Input: part model. Units: mm. Frame: model coordinates. Face numbers are marked on the shaded views. Coordinates: 2 decimals unless noted, no trailing zeros. Use a Markdown table: item, result. Add a question column.
1. Line query: L1, parallel to Y at x = 109.5, z = 121.5; L2, parallel to Z at x = 321.5, y = 302; L3, parallel to X at y = 96.5, z = 97.5. Output: solid intervals per line, ascending. Write a range as [from, to].
2. Draft query along Y for the marked faces 1, 2 and 3. Return one class per face: +Y half, -Y half, draft (parallel to the pull), parting line (faces both ways), or undercut.
3. Pin query (flat end, axial travel): pin 1 (8 mm diameter, centred on x = 297.5, z = 66.5, fed in from -Y); pin 2 (1 mm diameter, centred on y = 116, z = 108, fed in from +X). Return the tip coordinate at first contact, or that it passes through.
```python
from build123d import *

# Parameters (mm, degrees)
F0_W     = 508
F0_H     = 381
F1_DEPTH = 127
F2_W     = 381
F2_H     = 254
F3_DEPTH = 38.1
F5_DEPTH = 127.001


with BuildPart() as f1:
    # F0 (on Top) → F1 (new body)
    with BuildSketch(Plane.XY):
        with Locations((254, 190.5)):
            Rectangle(F0_W, F0_H)
    extrude(amount=F1_DEPTH)

    # F2 (on face) → F3 (cut)
    with BuildSketch(Plane.XY.offset(127)):
        with Locations((254, 190.5)):
            Rectangle(F2_W, F2_H)
    extrude(amount=-F3_DEPTH, mode=Mode.SUBTRACT)

    # F4 (on face) → F5 (cut, through all)
    with BuildSketch(Plane.XY.offset(127)):
        with BuildLine():
            Line((444.5, 317.5), (384.4547422164, 317.5))
            add(Edge.make_bspline(
                [(93.5035740318, 63.5), (147.2071592582, 101.4136170576), (240.8619840218, 173.7700888717), (344.3781582981, 281.8687103961), (384.4547422164, 317.4999999999)],
                knots=[0.1203807823, 0.1203807823, 0.1203807823, 0.1203807823, 0.3259105165, 0.4706282149, 0.4706282149, 0.4706282149, 0.4706282149], degree=3))
            Line((93.5035740318, 63.5), (444.5, 63.5))
            Line((444.5, 63.5), (444.5, 317.5))
        make_face()
        with BuildLine():
            Line((508, 0), (508, 381))
            Line((508, 381), (484.2276728464, 381))
            add(Edge.make_bspline(
                [(384.4547422164, 317.4999999999), (421.0763564574, 350.0595451308), (455.4476445846, 375.0758613525), (484.2276728464, 381)],
                knots=[0.4706282149, 0.4706282149, 0.4706282149, 0.4706282149, 0.6028699184, 0.6028699184, 0.6028699184, 0.6028699184], degree=3))
            Line((384.4547422164, 317.5), (444.5, 317.5))
            Line((444.5, 317.5), (444.5, 63.5))
            Line((444.5, 63.5), (93.5035740318, 63.5))
            add(Edge.make_bspline(
                [(0, 0), (31.0244285766, 20.6468112151), (62.0488571531, 41.2936224301), (93.5035740318, 63.5)],
                knots=[0, 0, 0, 0, 0.1203807823, 0.1203807823, 0.1203807823, 0.1203807823], degree=3))
            Line((0, 0), (508, 0))
        make_face()
        with BuildLine():
            add(Edge.make_bspline(
                [(508, 381), (576.339941908, 364.0495678727), (596.4256136065, 182.0247839364), (616.511285305, 0)],
                knots=[0.6416145202, 0.6416145202, 0.6416145202, 0.6416145202, 1, 1, 1, 1], degree=3))
            Line((508, 381), (508, 0))
            Line((508, 0), (616.511285305, 0))
        make_face()
    extrude(amount=-F5_DEPTH, mode=Mode.SUBTRACT)


solid = f1.part
```
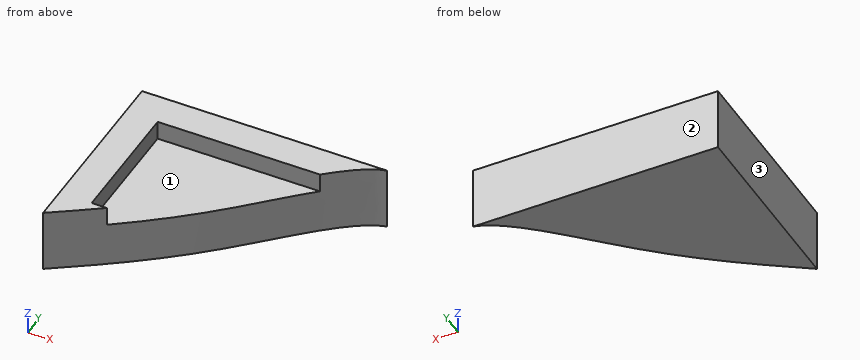
Answers below:
| question | item | result |
|---|---|---|
| 1 | L1 | y = [317.5, 381] |
| 1 | L2 | z = [0, 88.9] |
| 1 | L3 | x = [0, 63.5] |
| 2 | face 1 | undercut |
| 2 | face 2 | +Y half |
| 2 | face 3 | draft |
| 3 | pin 1 | stops at y = 230.34 |
| 3 | pin 2 | stops at x = 63.5 |
